from build123d import *

# Parameters (mm, degrees)
BOSS_EXTRUDE1_DEPTH = 4
FILLET1_R           = 4
FILLET2_R           = 2


with BuildPart() as part:
    # Sketch1 → Boss-Extrude1 (new body)
    with BuildSketch(Plane.XY):
        with BuildLine():
            Line((0, 0), (0, 2.5))
            Line((0, 2.5), (20, 2.5))
            Line((20, 2.5), (20, 7))
            Line((20, 7), (0, 7))
            ThreePointArc((0, 7), (-47.899542657, 25.027060394), (-68, 72.09416895))
            Line((-68, 72.09416895), (-68, 121.5))
            Line((-68, 121.5), (20, 121.5))
            Line((20, 121.5), (20, 125.5))
            Line((20, 125.5), (0, 125.5))
            Line((0, 125.5), (0, 128))
            ThreePointArc((0, 128), (-6.772700236, 126.180912146), (-13.752306798, 125.5))
            Line((-13.752306798, 125.5), (-68, 125.5))
            Line((-68, 125.5), (-72, 125.5))
            Line((-72, 125.5), (-72, 72.09416895))
            ThreePointArc((-72, 72.09416895), (-51.025872308, 21.040838867), (0, 0))
        make_face()
    extrude(amount=BOSS_EXTRUDE1_DEPTH)

    # Fillet1
    fillet1_edges = [part.edges().sort_by_distance(p)[0] for p in [
        (-68, 121.5, 2),
    ]]
    fillet(fillet1_edges, radius=FILLET1_R)

    # Fillet2
    fillet2_edges = [part.edges().sort_by_distance(p)[0] for p in [
        (-72, 125.5, 2),
    ]]
    fillet(fillet2_edges, radius=FILLET2_R)


solid = part.part
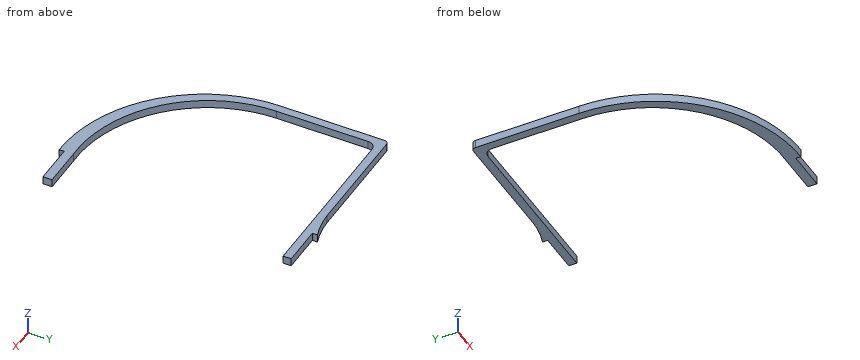
Could you check a few things on this model? Use its own coordinates, in mm. Give positions to 0.01 mm unless a question says otherwise; leave off trailing zeros. Order: outer loops, then holes, each group sorted by start corner. A loop starts at its lowest first (then second) coordinate and runs counter-clockwise, first axis right, second up. Notation, with made-up numbers: (-7.75, 2) - (38.25, 2) arc R21 cw to (38.25, 11) - close; hole circle Ø7 at (74.25, 56.25). An arc over 180 degrees is marked (long way). One line per question, with ' | ' between items. Start each with the question number.
Item 1: I want a section at B-B on z = 1.35. Write out the boundary of the cut face in (x, y), then the cut area to 3 significant figures.
Item 2: I'm going to push flat-ended pins straight in: pin 1 Ø1.2 at (x, z) = (10, 2.5) entering from -Y; pin 2 Ø0.8 at (y, z) = (1, 1.5) entering from +X; pin 3 Ø1.2 at (y, z) = (102.5, 1) entering from +X. Where does each tip first touch, or does it pass through?
Item 3: I want a section at D-D on y = 113. Write out the boundary of the cut face in (x, z), then the cut area to 3 significant figures.
Item 4: I need wall thicknesses on probe 1 along Y at (x, z) = (13.5, 0.9); probe 2 along X at (y, z) = (113.5, 1.45); probe 3 along Y at (x, z) = (-47, 3.65). Which ranges of each line are inside material? Lowest first, please. Write a range as [from, to].
Item 5: I want a section at C-C on x = -17. Write out the boundary of the cut face in (y, z), then the cut area to 3 significant figures.
Item 6: I want a section at A-A on x = 3. Write out the boundary of the cut face in (y, z), then the cut area to 3 significant figures.
Verdict:
1) outline: (-72, 72.09) arc R71.73 ccw to (0, 0) - (0, 2.5) - (20, 2.5) - (20, 7) - (0, 7) arc R65.16 cw to (-68, 72.09) - (-68, 117.5) arc R4 cw to (-64, 121.5) - (20, 121.5) - (20, 125.5) - (0, 125.5) - (0, 128) arc R42.51 cw to (-13.75, 125.5) - (-70, 125.5) arc R2 ccw to (-72, 123.5) - close | area: 1,240 mm^2
2) pin 1: y = 2.5 | pin 2: x = 0 | pin 3: x = -68
3) outline: (-72, 0) - (-68, 0) - (-68, 4) - (-72, 4) - close | area: 16.0 mm^2
4) probe 1: [2.5, 7], [121.5, 125.5] | probe 2: [-72, -68] | probe 3: [17.31, 24.18], [121.5, 125.5]
5) outline: (1.98, 0) - (8.49, 0) - (8.49, 4) - (1.98, 4) - close; (121.5, 0) - (125.5, 0) - (125.5, 4) - (121.5, 4) - close | area: 42.1 mm^2
6) outline: (2.5, 0) - (7, 0) - (7, 4) - (2.5, 4) - close; (121.5, 0) - (125.5, 0) - (125.5, 4) - (121.5, 4) - close | area: 34.0 mm^2
